Read the model definition and answer for the solid it produces. Units are mm, in the model's axes. Face numbers are marked on the shaded views. A direction names the side the tool comes from. Coordinates: 2 decimals unless noted, no trailing zeros. Order: outer loops, then holes, each group sorted by start corner. A loop starts at its lowest first (then second) coordinate and runs counter-clockwise, first axis right, second up. Notation, with made-up numbers: (-37.75, 76.25) -> (21.25, 76.25) arc R26 ccw to (21.25, 111.25) -> close; hole circle Ø10 at (48, -5.5). An arc over 180 degrees is marked (long way). Answer in a Markdown table with one row per item.
from build123d import *

# Parameters (mm, degrees)
SKETCH_1_R      = 1.55
SKETCH_1_W      = 7.455
SKETCH_1_H      = 15
EXTRUDE_1_DEPTH = 3
FILLET_1_R      = 2
FILLET_2_R      = 1


with BuildPart() as part:
    # 草图1 → 凸台-拉伸1 (new body)
    with BuildSketch(Plane.XY):
        with BuildLine():
            Line((-13, 14.5), (-13, 11.5))
            ThreePointArc((-13, 11.5), (-14.005, 10.495), (-15.01, 11.5))
            Line((-15.01, 11.5), (-23.455, 11.5))
            Line((-23.455, 11.5), (-23.455, -11.5))
            Line((-23.455, -11.5), (-15.01, -11.5))
            ThreePointArc((-15.01, -11.5), (-14.005, -10.495), (-13, -11.5))
            Line((-13, -11.5), (-13, -14.5))
            Line((-13, -14.5), (-7, -14.5))
            Line((-7, -14.5), (-7, -11.5))
            ThreePointArc((-7, -11.5), (-5.995, -10.495), (-4.99, -11.5))
            Line((-4.99, -11.5), (23.455, -11.5))
            Line((23.455, -11.5), (23.455, 11.5))
            Line((23.455, 11.5), (-4.99, 11.5))
            ThreePointArc((-4.99, 11.5), (-5.995, 10.495), (-7, 11.5))
            Line((-7, 11.5), (-7, 14.5))
            Line((-7, 14.5), (-13, 14.5))
        make_face()
        with Locations((-20.455, -8)):
            Circle(SKETCH_1_R, mode=Mode.SUBTRACT)
        with Locations((20.455, -8)):
            Circle(SKETCH_1_R, mode=Mode.SUBTRACT)
        Polygon((9.2275, -2.161680579), (14.371860482, -7.5), (4.083139518, -7.5), align=None, mode=Mode.SUBTRACT)
        with Locations((-12.7275, 0)):
            Rectangle(SKETCH_1_W, SKETCH_1_H, mode=Mode.SUBTRACT)
        with BuildLine():
            ThreePointArc((-0.995, -3.995), (-1.289357685, -4.705642315), (-2, -5))
            Line((-2, -5), (-5, -5))
            ThreePointArc((-5, -5), (-6.005, -3.995), (-5, -2.99))
            Line((-5, -2.99), (-5, 2.99))
            ThreePointArc((-5, 2.99), (-6.005, 3.995), (-5, 5))
            Line((-5, 5), (-2, 5))
            ThreePointArc((-2, 5), (-1.289357685, 4.705642315), (-0.995, 3.995))
            ThreePointArc((-0.995, 3.995), (-1.289357685, 3.284357685), (-2, 2.99))
            Line((-2, 2.99), (-2, -2.99))
            ThreePointArc((-2, -2.99), (-1.289357685, -3.284357685), (-0.995, -3.995))
        make_face(mode=Mode.SUBTRACT)
        with Locations((-20.455, 8)):
            Circle(SKETCH_1_R, mode=Mode.SUBTRACT)
        Polygon((2, -5.338319421), (2, 5.338319421), (7.144360482, 0), align=None, mode=Mode.SUBTRACT)
        Polygon((4.083139518, 7.5), (14.371860482, 7.5), (9.2275, 2.161680579), align=None, mode=Mode.SUBTRACT)
        Polygon((11.310639518, 0), (16.455, 5.338319421), (16.455, -5.338319421), align=None, mode=Mode.SUBTRACT)
        with Locations((20.455, 8)):
            Circle(SKETCH_1_R, mode=Mode.SUBTRACT)
    extrude(amount=EXTRUDE_1_DEPTH)

    # 圆角1
    fillet_1_edges = [part.edges().sort_by_distance(p)[0] for p in [
        (-23.455, -11.5, 1.5),
        (-23.455, 11.5, 1.5),
        (23.455, 11.5, 1.5),
        (23.455, -11.5, 1.5),
        (-16.455, -7.5, 1.5),
        (-9, -7.5, 1.5),
        (-9, 7.5, 1.5),
        (-16.455, 7.5, 1.5),
    ]]
    fillet(fillet_1_edges, radius=FILLET_1_R)

    # 圆角2
    fillet_2_edges = [part.edges().sort_by_distance(p)[0] for p in [
        (16.455, -5.338319421, 1.5),
        (16.455, 5.338319421, 1.5),
        (11.310639518, 0, 1.5),
        (14.371860482, -7.5, 1.5),
        (9.2275, -2.161680579, 1.5),
        (4.083139518, -7.5, 1.5),
        (2, 5.338319421, 1.5),
        (2, -5.338319421, 1.5),
        (7.144360482, 0, 1.5),
        (14.371860482, 7.5, 1.5),
        (4.083139518, 7.5, 1.5),
        (9.2275, 2.161680579, 1.5),
    ]]
    fillet(fillet_2_edges, radius=FILLET_2_R)


solid = part.part
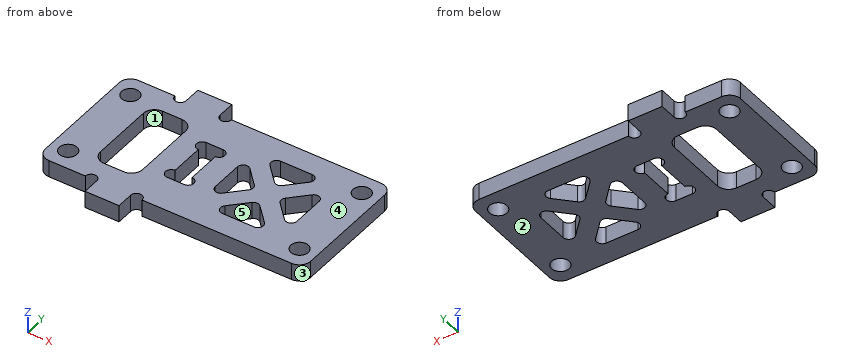
Q1. Consider line 1 (Y direction, x = -20.5, z = 1.2); line 2 (Y direction, x = 15.5, z = 0.45); line 3 (X direction, y = 4, z = 2.25) (3 decimals). Determine where each line is inside the solid, lowest interval first.
Outcome:
| item | result |
|---|---|
| line 1 | -11.5 to -9.55, -6.45 to 6.45, 9.55 to 11.5 |
| line 2 | -11.5 to -3.86, 3.86 to 11.5 |
| line 3 | -23.455 to -16.455, -9 to -6.005, -0.995 to 7.456, 10.999 to 23.455 |
Q2. Given pin 1 (1.5 mm diameter, centred on y = 13.5, z = 2, fed in from +X); pin 2 (1.5 mm diameter, centred on x = -18, z = 1.5, fed in from +Y); pin 3 (12 mm diameter, centred on x = -12.5, y = -2.5, fed in from -Z); pin 4 (1.5 mm diameter, centred on y = -10.5, z = 1.5, fed in from +X), each flat-ended and moving along its own axis, determine where each tip first touches the part or whether it passes through.
Outcome:
| item | result |
|---|---|
| pin 1 | x = -7 |
| pin 2 | y = 11.5 |
| pin 3 | z = 0 |
| pin 4 | x = 23.44 |
Q3. For the marked faces 1 and 2, determine the directions among +Z, -Z, +X, -X, +Y, -Y from which every point of the face is accessible in a straight line to the end or side of a thin tool.
Outcome:
| item | result |
|---|---|
| face 1 | +Z, -Z |
| face 2 | -Z, +X, -X, +Y, -Y |
Q4. The part is cut by section A-A (y = -8). Write down the section's boundary in (x, z) (3 decimals).
Outcome:
| item | result |
|---|---|
| outline | (-23.455, 0) -> (-22.005, 0) -> (-22.005, 3) -> (-23.455, 3) -> close; (-18.905, 0) -> (18.905, 0) -> (18.905, 3) -> (-18.905, 3) -> close; (22.005, 0) -> (23.455, 0) -> (23.455, 3) -> (22.005, 3) -> close |
Q5. The part is cut by section D-D (z = 1.95). Give the number of separate pieces and of enclosed holes in the cut face, then the cut area to 3 significant figures.
Outcome:
| item | result |
|---|---|
| separate pieces | 1 |
| enclosed holes | 10 |
| area | 831 mm² |
Q6. For a pull along Y with two mould halves and no side action, classify the marked faces 3, 4 and 5 as pulls with the +Y half, pulls with the -Y half, needs draft (parallel to the pull), parting line crosses it, or undercut.
Outcome:
| item | result |
|---|---|
| face 3 | pulls with the -Y half |
| face 4 | needs draft |
| face 5 | undercut |
Q7. The part is cut by section B-B (x = -4.5). Write down the section's boundary in (y, z).
Outcome:
| item | result |
|---|---|
| outline | (-11.5, 0) -> (-5, 0) -> (-5, 3) -> (-11.5, 3) -> close; (5, 0) -> (11.5, 0) -> (11.5, 3) -> (5, 3) -> close |
Q8. The part is cut by section C-C (y = 2). Write down the section's boundary in (x, z) (3 decimals).
Outcome:
| item | result |
|---|---|
| outline | (-23.455, 0) -> (-16.455, 0) -> (-16.455, 3) -> (-23.455, 3) -> close; (-9, 0) -> (-5, 0) -> (-5, 3) -> (-9, 3) -> close; (-2, 0) -> (2, 0) -> (2, 3) -> (-2, 3) -> close; (5.217, 0) -> (13.238, 0) -> (13.238, 3) -> (5.217, 3) -> close; (16.455, 0) -> (23.455, 0) -> (23.455, 3) -> (16.455, 3) -> close |
